Here's how the part is built. I have some questions about the finished solid (model axes, mm). Coordinates: 2 decimals unless noted, no trailing zeros. Order: outer loops, then holes, each group sorted by start corner. A loop starts at its lowest first (then second) coordinate and runs counter-clockwise, first axis right, second up.
Autodesk Inventor part; units mm, degrees
ref_plane "YZ Plane" through (0, 0, 0) normal (1, 0, 0) x (0, 1, 0)
ref_plane "XZ Plane" through (0, 0, 0) normal (0, 1, 0) x (-1, 0, 0)
ref_plane "XY Plane" through (0, 0, 0) normal (0, 0, 1) x (1, 0, 0)
sketch "Sketch1" plane through (0, 0, 0) normal (0, 0, 1) x (1, 0, 0)
  line L0 (140, 5) -> (-140, 5)
  line L1 (-140, 5) -> (-140, -5)
  line L2 (-140, -5) -> (140, -5)
  line L3 (140, -5) -> (140, 5)
  line L4 (140, 5) -> (-140, -5) construction
  line L5 (-140, 5) -> (140, -5) construction
  point P0 (0, 0)
  dimension "d0" = 280
  dimension "d1" = 10
extrude "Extrusion1" add sketch "Sketch1" along normal blind 20
sketch "Sketch3" plane through (-140, -5, 0) normal (-1, 0, 0) x (0, 0, 1)
  line L0 (0, 10) -> (0, 0)
  line L1 (20, 10) -> (20, 0)
  line L2 (0, 10) -> (20, 0)
  line L3 (20, 0) -> (20, 10)
  line L4 (0, 10) -> (20, 10)
  line L5 (20, 10) -> (0, 10)
  point P0 (0, 5)
extrude "Extrusion3" cut sketch "Sketch3" against normal through all
sketch "Sketch5" plane through (-140, -5, 0) normal (0, -1, 0) x (1, 0, 0)
  circle A0 centre (37.5, 12) radius 2
  circle A1 centre (233.5, 12) radius 2
  line L0 (0, 20) -> (280, 20)
  line L1 (0, 0) -> (0, 20)
  point P0 (140, 0)
  dimension "d8" = 4
  dimension "d9" = 4
  dimension "d10" = 196
  dimension "d11" = 8
  dimension "d12" = 8
  dimension "d13" = 37.5
hole "Hole1" at (93.5, -5, 12) at (-102.5, -5, 12) direction (0, 1, 0) diameter 4 depth 5 tip angle 118
properties part number "paw shelf_v01"
Q1. If we section it at C-C on z = 17.5: Write out the boundary of the cut face in (x, y), then the cut area to 3 significant figures.
Q2. I need wall thicknesses on L1, parallel to X at y = -2.35, z = 12; L2, parallel to Z at x = 93.5, y = -3; L3, parallel to Z at x = 93.5, y = -1.6. Which ranges of each line are inside material? Lowest first, please.
Q3. If we section it at A-A on x = -32: Write out the boundary of the cut face in (y, z), then the cut area to 3 significant figures.
Q4. Will these pins go through, and if not, where does the flat tip stop? pin 1 (5 mm diameter, centred on x = 71.5, y = -0.5, fed in from +Z); pin 2 (5 mm diameter, centred on x = -78.5, z = 6.5, fed in from +Y); pin 3 (3 mm diameter, centred on x = 54, y = -0.5, fed in from -Z).
Q5. If we section it at B-B on z = 6.5: Write out the boundary of the cut face in (x, y), then the cut area to 3 significant figures.
Reply:
1. outline: (-140, -5) - (140, -5) - (140, -3.75) - (-140, -3.75) - close
1. area: 350 mm2
2. L1: x = -140 to -104.5, -100.5 to 91.5, 95.5 to 140
2. L2: z = 0 to 10, 14 to 16
2. L3: z = 0 to 10
3. outline: (-5, 0) - (5, 0) - (-5, 20) - close
3. area: 100 mm2
4. pin 1: stops at z = 16
4. pin 2: stops at y = 3
4. pin 3: stops at z = 0
5. outline: (-140, -5) - (140, -5) - (140, 1.75) - (-140, 1.75) - close
5. area: 1,890 mm2
